```python
from build123d import *

# Parameters (mm, degrees)
SKETCH8_R      = 6.35
EXTRUDE1_DEPTH = 97.79


with BuildPart() as part:
    # Sketch1 → Revolve1 (revolve)
    with BuildSketch(Plane.XY, mode=Mode.PRIVATE) as revolve1_sk:
        Polygon((-48.22399997, 35.097050796), (-40.462, 35.097050796), (-40.462, 38.978050908), (-32.7, 38.978050908), (-32.7, 35.097050796), (-32.7, 11.811050572), (-71.50999988, 11.811050572), (-71.50999988, 23.454050572), (-63.74799991, 23.454050572), (-63.74799991, 27.335050572), (-55.98599994, 27.335050572), (-55.98599994, 31.216050684), (-48.22399997, 31.216050684), align=None)
    revolve(revolve1_sk.sketch.rotate(Axis((0, 0, 0), (0, 1, 0)), 270), axis=Axis((0, 0, 0), (0, 1, 0)))

    # Sketch8 → Extrude1 (add)
    with BuildSketch(Plane(origin=(0, 23.454050572, 0), x_dir=(1, 0, 0), z_dir=(0, 1, 0))):
        with Locations(Location((-58.42, 0, 0), (0, 0, 64.553386738))):
            Circle(SKETCH8_R)
        with Locations(Location((58.42, 0, 0), (0, 0, 90))):
            Circle(SKETCH8_R)
        with Locations(Location((0, 58.42, 0), (0, 0, 55.38310385))):
            Circle(SKETCH8_R)
    extrude(amount=EXTRUDE1_DEPTH)


solid = part.part
```
CAD build for the part. Positions are in the model's coordinates, mm. A direction names the side the tool comes from. Round coordinates to 2 decimals unless told otherwise and drop trailing zeros. Order: outer loops, then holes, each group sorted by start corner. A loop starts at its lowest first (then second) coordinate and runs counter-clockwise, first axis right, second up.
Item 1: Saw through at C-C on y = 71.5. Write the cut outline in (x, z), then the cut area to 3 significant figures.
Item 2: Probe line 1 along X through (y, z) = (30.75, 0); line 2 along Y through (x, z) = (41.5, 43.5); line 3 along X through (y, z) = (21, 0). List the from-to ranges inside material, lowest first.
Item 3: Saw through at A-A on z = 0. Write the cut outline in (x, y), then the cut area to 3 significant figures.
Item 4: Saw through at B-B on x = 0. Write the cut outline in (y, z).
Item 5: Mould opens along X. For faces 1 (the face through (-44.614, 25.422, -45.534)), 2 (the face through (40, 27.335, -40)), 3 (the face through (12.52, 25.58, -30.21)), 4 (the face through (-1.351, 25.422, 63.734)) say: pulls with the +X half, pulls with the -X half, needs draft (parallel to the pull), parting line crosses it, or undercut.
Item 6: Pin check, flat tip, straight feed: pin 1 (12 mm diameter, centred on x = 3.5, z = -31, fed in from +Y). Stop position of the tip, or through.
Item 7: Tool access for faces 5 (the face through (45.534, 25.422, -44.614)), 6 (the face through (0, 38.978, -33)), 7 (the face through (-2.47, 71.66, -64.27)): list every direction of +Z, -Z, +X, -X, +Y, -Y with a clear straight run to the whole face (end or side of a thin tool).
Item 8: Saw through at D-D on z = -58.42. Write the cut outline in (x, y).
Reported:
1. outline: circle Ø12.7 at (-58.42, 0); circle Ø12.7 at (0, -58.42); circle Ø12.7 at (58.42, 0)
1. area: 380 mm2
2. line 1: x = -64.77 to -32.7, 32.7 to 64.77
2. line 2: y = 11.81 to 27.34
2. line 3: x = -71.51 to -32.7, 32.7 to 71.51
3. outline: (-71.51, 11.81) - (-32.7, 11.81) - (-32.7, 38.98) - (-40.46, 38.98) - (-40.46, 35.1) - (-48.22, 35.1) - (-48.22, 31.22) - (-52.07, 31.22) - (-52.07, 121.24) - (-64.77, 121.24) - (-64.77, 23.45) - (-71.51, 23.45) - close; (32.7, 11.81) - (71.51, 11.81) - (71.51, 23.45) - (64.77, 23.45) - (64.77, 121.24) - (52.07, 121.24) - (52.07, 31.22) - (48.22, 31.22) - (48.22, 35.1) - (40.46, 35.1) - (40.46, 38.98) - (32.7, 38.98) - close
3. area: 3,870 mm2
4. outline: (11.81, -71.51) - (23.45, -71.51) - (23.45, -64.77) - (121.24, -64.77) - (121.24, -52.07) - (31.22, -52.07) - (31.22, -48.22) - (35.1, -48.22) - (35.1, -40.46) - (38.98, -40.46) - (38.98, -32.7) - (11.81, -32.7) - close; (11.81, 32.7) - (38.98, 32.7) - (38.98, 40.46) - (35.1, 40.46) - (35.1, 48.22) - (31.22, 48.22) - (31.22, 55.99) - (27.34, 55.99) - (27.34, 63.75) - (23.45, 63.75) - (23.45, 71.51) - (11.81, 71.51) - close
5. face 1: pulls with the -X half
5. face 2: needs draft
5. face 3: undercut
5. face 4: parting line crosses it
6. pin 1: stops at y = 38.98
7. face 5: -Z, +X, +Y
7. face 6: +Z, +Y
7. face 7: +Y
8. outline: (-41.24, 11.81) - (41.24, 11.81) - (41.24, 23.45) - (25.51, 23.45) - (25.51, 27.34) - (6.35, 27.34) - (6.35, 121.24) - (-6.35, 121.24) - (-6.35, 27.34) - (-25.51, 27.34) - (-25.51, 23.45) - (-41.24, 23.45) - close
